from build123d import *

# Parameters (mm, degrees)
SKETCH2_W                                  = 160
SKETCH2_H                                  = 160
OUTER_BLOCK_DEPTH                          = 35
SKETCH12_W                                 = 154
SKETCH12_H                                 = 154
CUT_EXTRUDE1_DEPTH                         = 6.5
SKETCH14_W                                 = 154
SKETCH14_H                                 = 154
CUT_EXTRUDE4_DEPTH                         = 20
SKETCH15_W                                 = 148
SKETCH15_H                                 = 148
CUT_EXTRUDE6_DEPTH                         = 7.5
SKETCH17_R                                 = 4
BOSS_EXTRUDE1_DEPTH                        = 5
MIRROR1_AT_THE_SECOND_PLANE_COPY_1_SKETC_R = 4
MIRROR1_AT_THE_SECOND_PLANE_COPY_1_DEPTH   = 5


with BuildPart() as part:
    # Sketch2 → Outer Block (new body)
    with BuildSketch(Plane(origin=(0, 0, 0), x_dir=(1, 0, 0), z_dir=(0, 1, 0))):
        Rectangle(SKETCH2_W, SKETCH2_H)
    extrude(amount=OUTER_BLOCK_DEPTH)

    # Sketch12 → Cut-Extrude1 (cut)
    with BuildSketch(Plane(origin=(0, 35, 0), x_dir=(1, 0, 0), z_dir=(0, 1, 0))):
        Rectangle(SKETCH12_W, SKETCH12_H)
    extrude(amount=-CUT_EXTRUDE1_DEPTH, mode=Mode.SUBTRACT)

    # Sketch14 → Cut-Extrude4 (cut)
    with BuildSketch(Plane(origin=(0, 3, 0), x_dir=(-1, 0, 0), z_dir=(0, -1, 0))):
        Rectangle(SKETCH14_W, SKETCH14_H)
    extrude(amount=-CUT_EXTRUDE4_DEPTH, mode=Mode.SUBTRACT)

    # Sketch15 → Cut-Extrude6 (cut)
    with BuildSketch(Plane(origin=(0, 28.5, 0), x_dir=(1, 0, 0), z_dir=(0, 1, 0))):
        Rectangle(SKETCH15_W, SKETCH15_H)
    extrude(amount=-CUT_EXTRUDE6_DEPTH, mode=Mode.SUBTRACT)

    # Sketch17 → Boss-Extrude1 (add)
    with BuildSketch(Plane.XZ):
        with Locations((-72.928932188, 72.928932188)):
            Circle(SKETCH17_R)
    boss_extrude1 = extrude(amount=BOSS_EXTRUDE1_DEPTH)

    # Mirror1: Boss-Extrude1 across plane
    add(boss_extrude1.mirror(Plane.XY))

    # Mirror1 at the second plane: Boss-Extrude1 across plane
    add(boss_extrude1.mirror(Plane(origin=(0, 0, 0), x_dir=(0, 0, 1), z_dir=(1, 0, 0))))

    # Mirror1 at the second plane copy 1 sketc → Mirror1 at the second plane copy 1 (add)
    with BuildSketch(Plane(origin=(0, 0, 0), x_dir=(-1, 0, 0), z_dir=(0, -1, 0))):
        with Locations((-72.928932188, 72.928932188)):
            Circle(MIRROR1_AT_THE_SECOND_PLANE_COPY_1_SKETC_R)
    extrude(amount=MIRROR1_AT_THE_SECOND_PLANE_COPY_1_DEPTH)


solid = part.part
Build history of the part. All positions in model axes, mm. A direction names the side the tool comes from. Give positions to 0.01 mm unless a question says otherwise; leave off trailing zeros. Order: outer loops, then holes, each group sorted by start corner. A loop starts at its lowest first (then second) coordinate and runs counter-clockwise, first axis right, second up. Notation, with made-up numbers: M 73,77.25 L 119,77.25 A18 cw 119,87.25 Z; hole C 58.25,38 d1. An arc over 180 degrees is marked long. Use one line per item in the form item = value.
1) Saw through at C-C (x = -10). Give the cut face in (y, z).
Calculated:
outline = M 0,-80 L 35,-80 L 35,-77 L 28.5,-77 L 28.5,-74 L 23,-74 L 23,-77 L 3,-77 L 3,77 L 23,77 L 23,74 L 28.5,74 L 28.5,77 L 35,77 L 35,80 L 0,80 Z
2) Tool access for faces 1 (the face through (1, 13, -77)), 2 (the face through (77, 32, 1)), 3 (the face through (-1, 0, -1)), 4 (the face through (-1, 17, 80)), 5 (the face through (-73, -5, -73)): list every direction of +Z, -Z, +X, -X, +Y, -Y with a clear straight run to the whole face (end or side of a thin tool).
Calculated:
face_1 = none
face_2 = +Y
face_3 = -Y
face_4 = +Z, +X, -X, +Y, -Y
face_5 = +Z, -Z, +X, -X, -Y
3) Saw through at A-A (z = -16). Give the cut face in (x, y), plus the area to 3 significant figures.
Calculated:
outline = M -80,0 L 80,0 L 80,35 L 77,35 L 77,28.5 L 74,28.5 L 74,23 L 77,23 L 77,3 L -77,3 L -77,23 L -74,23 L -74,28.5 L -77,28.5 L -77,35 L -80,35 Z
area = 705 mm2
4) Drop flat-ended pins along their axis: pin 1 (1.5 mm diameter, centred on x = -40.5, z = -22, fed in from -Y); pin 2 (3 mm diameter, centred on x = 53, z = -31.5, fed in from +Y). Give the stop position or say it passes through.
Calculated:
pin_1 = 0
pin_2 = 3
5) Saw through at B-B (y = 14.5). Give the cut face in (x, z).
Calculated:
outline = M -80,-80 L 80,-80 L 80,80 L -80,80 Z; hole M -77,-77 L 77,-77 L 77,77 L -77,77 Z
6) Probe probe 1 along X at (y, z) = (11, -41); probe 2 along X at (y, z) = (26.5, -21.5). List the from-to ranges inside material, lowest first.
Calculated:
probe_1 = -80 to -77, 77 to 80
probe_2 = -80 to -74, 74 to 80
7) Two-plate mould, pull along Y, no slides. Class faces 6 (the face through (73, -5, -73)), 7 (the face through (-80, 17, 1)), 8 (the face through (1, 13, 77)): released by +Y, released by -Y, zero draft, split by the parting line, or undercut.
Calculated:
face_6 = released by -Y
face_7 = zero draft
face_8 = undercut
